Read the model definition and answer for the solid it produces. Units are mm, in the model's axes. Face numbers are marked on the shaded views. A direction names the side the tool comes from. Coordinates: 2 decimals unless noted, no trailing zeros. Loops run counter-clockwise (first coordinate to the right, second up) from the corner with the lowest first, then second, coordinate; pieces in that order, holes last.
Q1. Straight lines are drawn through the part: line 1 (Y direction, x = -2.5, z = -6.75); line 2 (Z direction, x = 2.75, y = 2.5); line 3 (X direction, y = 9.75, z = 3). For each, find the intervals that lie inside material, in ascending order.
Q2. Section A-A (x = 0) is taken. Give the vertices of the cut face in (y, z), then the cut area to 3 significant figures.
Q3. Section C-C (z = -1.5) is taken. Give the vertices of the cut face in (x, y).
Q4. Which of the six approach directions +Z, -Z, +X, -X, +Y, -Y give full straight-line access (tool end or side, diameter ignored) to the marked faces 5, 6, 7, 8 and 9?
Q5. Flat-ended cylindrical pins translate along their axes: P1, Ø9.5, axis at x = 0.5, y = 0, coming from the -Z side; P2, Ø1, axis at x = -9, z = 2.5, coming from the -Y side; P3, Ø6, axis at y = 3.5, z = -5, coming from the +X side; P4, Ø4.5, axis at y = 5.5, z = 4, coming from the +X side. Find the tip coordinate at first contact, or state that the pin passes through.
Q6. The mould has two halves that part along X. Classify the marked faces 1, 2, 3 and 4: pulls with the +X half, pulls with the -X half, needs draft (parallel to the pull), parting line crosses it, or undercut.
Q7. Section B-B (y = 10.75) is taken. Give the vertices of the cut face in (x, z), then the cut area to 3 significant figures.
Q8. Section D-D (y = 8) is taken. Give the vertices of the cut face in (x, z), then the cut area to 3 significant figures.
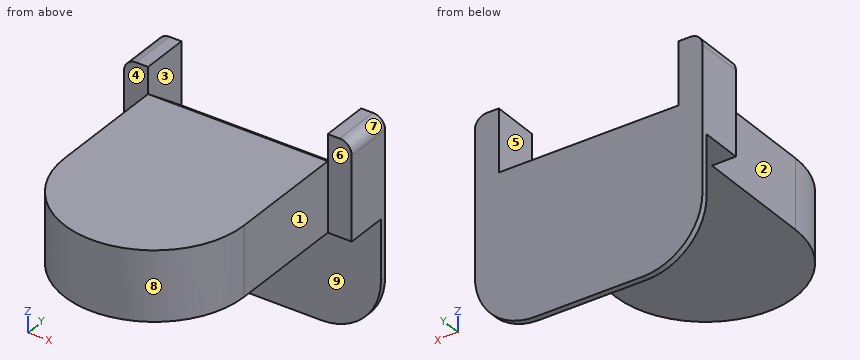
from build123d import *

# Parameters (mm, degrees)
F0_W     = 15
F0_H     = 0.5
F1_DEPTH = 5.8
F2_SIZE2 = 4
F2_SIZE  = 3
F0_W_2   = 2
F0_H_2   = 3.5
F3_DEPTH = 8
F4_DEPTH = 10
F5_R     = 1
F6_R     = 5


with BuildPart() as f1:
    # F0 (on Top) → F1 (new body)
    with BuildSketch(Plane.XY):
        with BuildLine():
            Line((-7.5, 10), (-7.5, 0))
            ThreePointArc((-7.5, 0), (0, -7.5), (7.5, 0))
            Line((7.5, 0), (7.5, 10))
            Line((7.5, 10), (7.5, 13.5))
            Line((7.5, 13.5), (-7.5, 13.5))
            Line((-7.5, 13.5), (-7.5, 10))
        make_face()
        with Locations((0, 13.75)):
            Rectangle(F0_W, F0_H)
    extrude(amount=F1_DEPTH)

    # F2
    f2_edges = [f1.edges().sort_by_distance(p)[0] for p in [
        (0, 14, 5.8),
    ]]
    chamfer(f2_edges, length=F2_SIZE, length2=F2_SIZE2)

    # F0 (on Top) → F3 (join)
    with BuildSketch(Plane.XY):
        with Locations((-8.5, 11.75)):
            Rectangle(F0_W_2, F0_H_2)
        with Locations((8.5, 13.75)):
            Rectangle(F0_W_2, F0_H)
        with Locations((8.5, 11.75)):
            Rectangle(F0_W_2, F0_H_2)
        with Locations((-8.5, 13.75)):
            Rectangle(F0_W_2, F0_H)
    extrude(amount=F3_DEPTH)

    # F0 (on Top) → F4 (join)
    with BuildSketch(Plane.XY):
        with Locations((0, 13.75)):
            Rectangle(F0_W, F0_H)
        with Locations((8.5, 13.75)):
            Rectangle(F0_W_2, F0_H)
        with Locations((-8.5, 13.75)):
            Rectangle(F0_W_2, F0_H)
    extrude(amount=-F4_DEPTH)

    # F5
    f5_edges = [f1.edges().sort_by_distance(p)[0] for p in [
        (-9.5, 12, 8),
        (9.5, 12, 8),
    ]]
    fillet(f5_edges, radius=F5_R)

    # F6
    f6_edges = [f1.edges().sort_by_distance(p)[0] for p in [
        (9.5, 13.75, -10),
        (-9.5, 13.75, -10),
    ]]
    fillet(f6_edges, radius=F6_R)


solid = f1.part
Numbers:
1. line 1: y = 13.5 to 14
1. line 2: z = 0 to 5.8
1. line 3: x = -7.5 to 7.5
2. outline: (-7.5, 0) - (13.5, 0) - (13.5, -10) - (14, -10) - (14, 2.8) - (10, 5.8) - (-7.5, 5.8) - close
2. area: 124 mm2
3. outline: (-9.5, 13.5) - (9.5, 13.5) - (9.5, 14) - (-9.5, 14) - close
4. face 5: +Z, +Y
4. face 6: +Z, -Z, +X, -Y
4. face 7: +Z, +X, +Y, -Y
4. face 8: +Z, -Z, -Y
4. face 9: -Z, +X, -X, -Y
5. P1: stops at z = 0
5. P2: stops at y = 10
5. P3: passes through
5. P4: stops at x = 7.5
6. face 1: pulls with the +X half
6. face 2: pulls with the -X half
6. face 3: undercut
6. face 4: needs draft
7. outline: (-9.5, 0) - (9.5, 0) - (9.5, 7) arc R1 ccw to (8.5, 8) - (7.5, 8) - (7.5, 5.24) - (-7.5, 5.24) - (-7.5, 8) - (-8.5, 8) arc R1 ccw to (-9.5, 7) - close
7. area: 110 mm2
8. outline: (-7.5, 0) - (7.5, 0) - (7.5, 5.8) - (-7.5, 5.8) - close
8. area: 87.0 mm2
